The listing builds one solid part. Answer for the finished solid, in the listing's coordinates (mm). Face numbers are marked on the shaded views. Give positions to 0.01 mm unless a question says otherwise; leave off trailing zeros. Loops run counter-clockwise (first coordinate to the right, second up) from the corner with the lowest first, then second, coordinate; pieces in that order, holes last. Notation, with made-up numbers: M 38,39.25 L 80,39.25 A24 ccw 80,52.25 Z; hole C 2.25,-7 d7. An arc over 180 degrees is marked long. Return JSON: item names as keys, results as strings.
from build123d import *

# Parameters (mm, degrees)
F0_R     = 4.69
F0_W     = 58.73
F0_H     = 103.15
F0_R_2   = 2.195
F0_R_3   = 1.058193308
F0_R_4   = 5.3501775611
F1_DEPTH = 7.08
F2_DEPTH = 7.08
F4_DEPTH = 0.8
F5_T     = 3


# Not quite as in the source:
# - a feature of the source that left no trace in its solid (it failed there, or was rolled back) is left out


with BuildPart() as f1:
    # F0 (on Front) → F1 (new body)
    with BuildSketch(Plane.XZ):
        with BuildLine():
            Line((23.565, 69.16), (-23.565, 69.16))
            ThreePointArc((-23.565, 69.16), (-30.6360678119, 66.2310678119), (-33.565, 59.16))
            Line((-33.565, 59.16), (-33.565, -59.16))
            ThreePointArc((-33.565, -59.16), (-30.6360678119, -66.2310678119), (-23.565, -69.16))
            Line((-23.565, -69.16), (23.565, -69.16))
            ThreePointArc((23.565, -69.16), (30.6360678119, -66.2310678119), (33.565, -59.16))
            Line((33.565, -59.16), (33.565, 59.16))
            ThreePointArc((33.565, 59.16), (30.6360678119, 66.2310678119), (23.565, 69.16))
        make_face()
        with Locations((0, -60.0285455585)):
            Circle(F0_R, mode=Mode.SUBTRACT)
        Rectangle(F0_W, F0_H, mode=Mode.SUBTRACT)
        with Locations((10.2654388174, 59.16)):
            Circle(F0_R_2, mode=Mode.SUBTRACT)
        with Locations((14.2954164479, 59.1465724891)):
            Circle(F0_R_3, mode=Mode.SUBTRACT)
        with Locations((21.3369000703, 59.16)):
            Circle(F0_R_4, mode=Mode.SUBTRACT)
        Rectangle(F0_W, F0_H)
        with Locations((21.3369000703, 59.16)):
            Circle(F0_R_4)
        with Locations((0, -60.0285455585)):
            Circle(F0_R)
        with Locations((10.2654388174, 59.16)):
            Circle(F0_R_2)
        with Locations((14.2954164479, 59.1465724891)):
            Circle(F0_R_3)
    extrude(amount=F1_DEPTH)

    # F0 (on Front) → F2 (join)
    with BuildSketch(Plane.XZ):
        Rectangle(F0_W, F0_H)
        with Locations((0, -60.0285455585)):
            Circle(F0_R)
    extrude(amount=F2_DEPTH)

    # F0 (on Front) → F4 (join)
    with BuildSketch(Plane.XZ):
        with Locations((21.3369000703, 59.16)):
            Circle(F0_R_4)
    extrude(amount=F4_DEPTH)

    # F5
    f5_openings = [f1.faces().sort_by_distance(p)[0] for p in [
        (0, -7.08, 0),
    ]]
    offset(amount=F5_T, openings=f5_openings, kind=Kind.INTERSECTION)


solid = f1.part
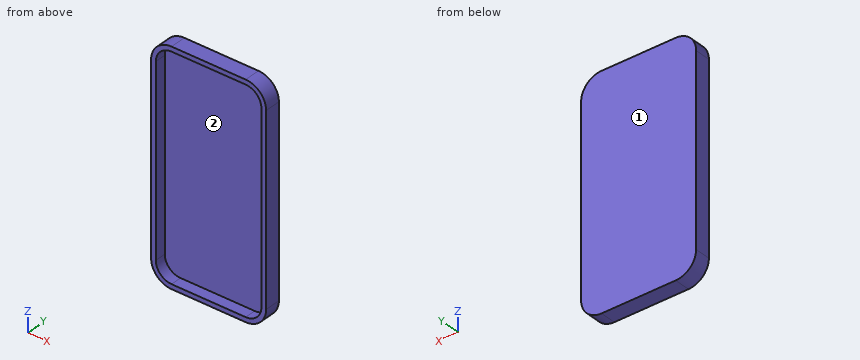
(1) Given pin 1 (3 mm diameter, centred on x = 1.5, z = -24.5, fed in from -Y), flat-ended and moving along its own axis, determine where the tip first touches the part or whether it passes through.
Values follow:
{"pin 1": "y = 0"}
(2) The part is cut by section B-B (y = -3.25). Determine the outline of the cut face in (x, z) (3 decimals), and give its area (3 significant figures).
Values follow:
{"outline": "M -36.565,-59.16 A13 ccw -23.565,-72.16 L 23.565,-72.16 A13 ccw 36.565,-59.16 L 36.565,59.16 A13 ccw 23.565,72.16 L -23.565,72.16 A13 ccw -36.565,59.16 Z; hole M -33.565,-59.16 A10 ccw -23.565,-69.16 L 23.565,-69.16 A10 ccw 33.565,-59.16 L 33.565,59.16 A10 ccw 23.565,69.16 L -23.565,69.16 A10 ccw -33.565,59.16 Z", "area": "1,210 mm²"}
(3) The part is cut by section C-C (z = -14). Determine the outline of the cut face in (x, y) (3 decimals).
Values follow:
{"outline": "M -36.565,-7.08 L -33.565,-7.08 L -33.565,0 L 33.565,0 L 33.565,-7.08 L 36.565,-7.08 L 36.565,3 L -36.565,3 Z"}
(4) Straight lines are drawn through the part: line 1 along X through (y, z) = (-3, 30) (3 decimals); line 2 along Z through (x, y) = (-4, -4.25); line 3 along Z through (x, y) = (24, -2.75). For each, find the intervals that lie inside material, in ascending order.
Values follow:
{"line 1": "-36.565 to -33.565, 33.565 to 36.565", "line 2": "-72.16 to -69.16, 69.16 to 72.16", "line 3": "-72.15 to -69.15, 69.15 to 72.15"}
(5) The part is cut by section A-A (x = -13). Determine the outline of the cut face in (y, z).
Values follow:
{"outline": "M -7.08,-72.16 L 3,-72.16 L 3,72.16 L -7.08,72.16 L -7.08,69.16 L 0,69.16 L 0,-69.16 L -7.08,-69.16 Z"}
(6) Determine the mould class of the marked faces 1 and 2 for opening direction X: released by +X, released by -X, zero draft, split by the parting line, or undercut.
Values follow:
{"face 1": "zero draft", "face 2": "undercut"}
